```python
from build123d import *

# Parameters (mm, degrees)
SKICA1_W                 = 160
SKICA1_H                 = 160
P_IDAT_VYSUNUT_M1_DEPTH  = 7
ODEBRAT_VYSUNUT_M1_DEPTH = 1
SKICA1_6_R               = 76
ODEBRAT_VYSUNUT_M3_DEPTH = 3


with BuildPart() as part:
    # Skica1 → P_idat vysunut_m1 (new body)
    with BuildSketch(Plane.XY):
        Rectangle(SKICA1_W, SKICA1_H)
    extrude(amount=P_IDAT_VYSUNUT_M1_DEPTH)

    # Skica1_5 → Odebrat vysunut_m1 (cut)
    with BuildSketch(Plane.XY):
        Polygon((-11, 27), (-11, 51), (11, 51), (11, 27), (27, 27), (27, 11), (51, 11), (51, -11), (27, -11), (27, -27), (11, -27), (11, -51), (-11, -51), (-11, -27), (-27, -27), (-27, -11), (-51, -11), (-51, 11), (-27, 11), (-27, 27), align=None)
    extrude(amount=ODEBRAT_VYSUNUT_M1_DEPTH, mode=Mode.SUBTRACT)

    # Skica1_6 → Odebrat vysunut_m3 (cut)
    with BuildSketch(Plane.XY):
        Circle(SKICA1_6_R)
        Polygon((-27, 27), (-11, 27), (-11, 51), (11, 51), (11, 27), (27, 27), (27, 11), (51, 11), (51, -11), (27, -11), (27, -27), (11, -27), (11, -51), (-11, -51), (-11, -27), (-27, -27), (-27, -11), (-51, -11), (-51, 11), (-27, 11), align=None, mode=Mode.SUBTRACT)
    extrude(amount=ODEBRAT_VYSUNUT_M3_DEPTH, mode=Mode.SUBTRACT)


solid = part.part
```
Could you check a few things on this model? Use its own coordinates, in mm. A direction names the side the tool comes from. Coordinates: 2 decimals unless noted, no trailing zeros. Write each loop counter-clockwise with the first axis right and the second up, starting at its lowest first coordinate (ties: lowest second). Pieces come first, ordered by that corner, then holes. Notation, with made-up numbers: M 15,-22 L 52,-22 A20 cw 52,-5 Z; hole C 80.25,-12.5 d1. An arc over 180 degrees is marked long. Answer as CSV lines item,"result". Start each with the question number.
1) Please list where these lines run through material, in increasing order: line 1 (Y direction, x = 0, z = 2); line 2 (Z direction, x = -27.5, y = -62); line 3 (Z direction, x = 7, y = 5). Write a range as from..to.
2) I want a section at C-C, the plane x = -58. Please give me the cut outline in (y, z), and give its area (3 significant figures).
3) For faces 1 (the flat face through (-1, 80, 3)), 2 (the cylindrical face through (35.069, -67.425, 1.479)), which set-ups out of +Z, -Z, +X, -X, +Y, -Y let a thin tool reach every point of the face, with its end or its side?
4) I want a section at D-D, the plane y = -56. Please give me the cut outline in (x, z), and give its area (3 significant figures).
5) I want a section at A-A, the plane x = 0. Please give me the cut outline in (y, z).
6) For P1, Ø5, axis at x = -10, y = -17, coming from the -Z side, with a flat end and sliding along its axis, tell me the tip position at first contact or that it passes through.
7) We'd pull the mould along X, two halves only. Please class faces 3 (the flat face through (1, 1, 1)), 4 (the flat face through (33, -16, 3)), 5 (the flat face through (-1, 1, 7)), 6 (the flat face through (-80, -1, 3)): +X half, -X half, draft (parallel to the pull), parting line (faces both ways), or undercut.
Data:
1,line 1,"y = -80..-76, -51..51, 76..80"
1,line 2,"z = 3..7"
1,line 3,"z = 1..7"
2,outline,"M -80,0 L -49.11,0 L -49.11,3 L 49.11,3 L 49.11,0 L 80,0 L 80,7 L -80,7 Z"
2,area,"825 mm^2"
3,face 1,"+Z, -Z, +X, -X, +Y"
3,face 2,"-Z"
4,outline,"M -80,0 L -51.38,0 L -51.38,3 L 51.38,3 L 51.38,0 L 80,0 L 80,7 L -80,7 Z"
4,area,"812 mm^2"
5,outline,"M -80,0 L -76,0 L -76,3 L -51,3 L -51,1 L 51,1 L 51,3 L 76,3 L 76,0 L 80,0 L 80,7 L -80,7 Z"
6,P1,"stops at z = 1"
7,face 3,"undercut"
7,face 4,"undercut"
7,face 5,"draft"
7,face 6,"-X half"
